Geometry: final body of the model. Coordinates: model frame, mm. Face numbers are marked on the shaded views. A direction names the side the tool comes from. Round coordinates to 2 decimals unless told otherwise and drop trailing zeros. Write each loop counter-clockwise with the first axis right and the second up, starting at its lowest first coordinate (ties: lowest second). Pieces come first, ordered by that corner, then holes. Notation, with made-up numbers: (-36.5, 81.25) -> (18.5, 81.25) arc R16 ccw to (18.5, 107.25) -> close; hole circle Ø7 at (61.5, -24). An arc over 180 degrees is marked (long way). One line per item, written item: value. Start each with the question number.
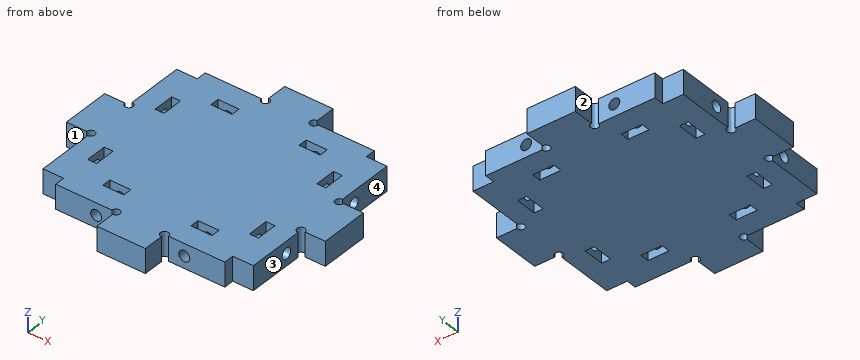
Autodesk Inventor part; units mm, degrees
ref_plane "YZ Plane" through (0, 0, 0) normal (1, 0, 0) x (0, 1, 0)
ref_plane "XZ Plane" through (0, 0, 0) normal (0, 1, 0) x (-1, 0, 0)
ref_plane "XY Plane" through (0, 0, 0) normal (0, 0, 1) x (1, 0, 0)
ref_plane "작업 평면1" through (0, 0, 0) normal (0, 0, 1) x (1, 0, 0)
sketch "스케치1" plane through (0, 0, 0) normal (0, 0, 1) x (1, 0, 0)
  line L0 (-18.9, 5.4) -> (-21.1, 5.4)
  line L1 (-21.1, 5.4) -> (-21.1, 10.6)
  line L2 (-21.1, 10.6) -> (-18.9, 10.6)
  line L3 (-18.9, 10.6) -> (-18.9, 5.4)
  line L4 (-21.1, -5.4) -> (-18.9, -5.4)
  line L5 (-18.9, -5.4) -> (-18.9, -10.6)
  line L6 (-18.9, -10.6) -> (-21.1, -10.6)
  line L7 (-21.1, -10.6) -> (-21.1, -5.4)
  line L8 (21.1, 5.4) -> (18.9, 5.4)
  line L9 (18.9, 5.4) -> (18.9, 10.6)
  line L10 (18.9, 10.6) -> (21.1, 10.6)
  line L11 (21.1, 10.6) -> (21.1, 5.4)
  line L12 (18.9, -10.6) -> (18.9, -5.4)
  line L13 (18.9, -5.4) -> (21.1, -5.4)
  line L14 (21.1, -5.4) -> (21.1, -10.6)
  line L15 (21.1, -10.6) -> (18.9, -10.6)
  circle A0 centre (8, -8) radius 1.35
  circle A1 centre (-8, 8) radius 1.35
  circle A2 centre (-8, -8) radius 1.35
  circle A3 centre (8, 8) radius 1.35
  line L16 (-26, 14) -> (-26, 3)
  line L17 (-26, 3) -> (-32, 3)
  line L18 (-32, 3) -> (-32, -3)
  line L19 (-32, -3) -> (-26, -3)
  line L20 (-26, -3) -> (-26, -14)
  line L21 (-26, -14) -> (26, -14)
  line L22 (26, -14) -> (26, -3)
  line L23 (26, -3) -> (32, -3)
  line L24 (32, -3) -> (32, 3)
  line L25 (32, 3) -> (26, 3)
  line L26 (26, 3) -> (26, 14)
  line L27 (26, 14) -> (-26, 14)
  line L28 (-11, -15.5) -> (-5, -15.5)
  line L29 (-5, -15.5) -> (-5, -18.5)
  line L30 (-5, -18.5) -> (-11, -18.5)
  line L31 (-11, -18.5) -> (-11, -15.5)
  line L32 (-5, 15.5) -> (-11, 15.5)
  line L33 (-11, 15.5) -> (-11, 18.5)
  line L34 (-11, 18.5) -> (-5, 18.5)
  line L35 (-5, 18.5) -> (-5, 15.5)
  line L36 (11, -18.5) -> (5, -18.5)
  line L37 (5, -18.5) -> (5, -15.5)
  line L38 (5, -15.5) -> (11, -15.5)
  line L39 (11, -15.5) -> (11, -18.5)
  line L40 (11, 15.0547) -> (5, 15.0547)
  line L41 (5, 15.0547) -> (5, 18.0547)
  line L42 (5, 18.0547) -> (11, 18.0547)
  line L43 (11, 18.0547) -> (11, 15.0547)
  circle A4 centre (8, 8) radius 1.35
  circle A5 centre (-8, -8) radius 1.35
  circle A6 centre (-8, 8) radius 1.35
  circle A7 centre (8, -8) radius 1.35
  line L44 (13.9, 23.5) -> (3, 23.5)
  line L45 (3, 23.5) -> (3, 29.5)
  line L46 (3, 29.5) -> (-3, 29.5)
  line L47 (-3, 29.5) -> (-3, 23.5)
  line L48 (-3, 23.5) -> (-13.9, 23.5)
  line L49 (-13.9, 23.5) -> (-13.9, -23.5)
  line L50 (-13.9, -23.5) -> (-3, -23.5)
  line L51 (-3, -23.5) -> (-3, -29.5)
  line L52 (-3, -29.5) -> (3, -29.5)
  line L53 (3, -29.5) -> (3, -23.5)
  line L54 (3, -23.5) -> (13.9, -23.5)
  line L55 (13.9, -23.5) -> (13.9, 23.5)
  line L56 (13.9, 23.5) -> (-13.9, 23.5)
  line L57 (-13.9, -23.5) -> (13.9, -23.5)
  line L58 (-26, 14) -> (-26, -14)
  line L59 (26, -14) -> (26, 14)
  line L60 (-26, -14) -> (-26, -21)
  line L61 (26, -21) -> (26, -14)
  line L62 (26, 14) -> (26, 21)
  line L63 (-26, 21) -> (-26, 14)
  line L64 (13.9, -23.5) -> (20.9, -23.5)
  line L65 (20.9, 23.5) -> (13.9, 23.5)
  line L66 (-13.9, 23.5) -> (-20.9, 23.5)
  line L67 (-20.9, -23.5) -> (-13.9, -23.5)
  line L68 (26, 21) -> (20.9, 21)
  line L69 (-20.9, 21) -> (-26, 21)
  line L70 (-20.9, -21) -> (-20.9, -23.5)
  line L71 (-20.9, 23.5) -> (-20.9, 21)
  line L72 (20.9, -23.5) -> (20.9, -21)
  line L73 (20.9, 21) -> (20.9, 23.5)
  line L74 (-26, -21) -> (-20.9, -21)
  line L75 (20.9, -21) -> (26, -21)
  line L76 (26, -5.994) -> (26, 6.006)
  line L77 (6, -23.5) -> (-6, -23.5)
  line L78 (-6, -23.5) -> (-6, -29.5)
  line L79 (-6, -29.5) -> (6, -29.5)
  line L80 (6, -29.5) -> (6, -23.5)
  line L81 (6, 23.5) -> (-6, 23.5)
  line L82 (-6, 23.5) -> (-6, 29.5)
  line L83 (-6, 29.5) -> (6, 29.5)
  line L84 (6, 29.5) -> (6, 23.5)
  line L85 (-26, 6) -> (-32, 6)
  line L86 (-32, 6) -> (-32, -6)
  line L87 (-32, -6) -> (-26, -6)
  line L88 (-26, -6) -> (-26, 6)
  line L89 (13.5, 18.1) -> (8.3, 18.1)
  line L90 (8.3, 18.1) -> (8.3, 15.9)
  line L91 (8.3, 15.9) -> (13.5, 15.9)
  line L92 (13.5, 15.9) -> (13.5, 18.1)
  line L93 (13.5, 18.1) -> (8.3, 15.9) construction
  line L94 (8.3, 18.1) -> (13.5, 15.9) construction
  line L95 (-13.5, 18.1) -> (-8.3, 18.1)
  line L96 (-8.3, 18.1) -> (-8.3, 15.9)
  line L97 (-8.3, 15.9) -> (-13.5, 15.9)
  line L98 (-13.5, 15.9) -> (-13.5, 18.1)
  line L99 (-13.5, 18.1) -> (-8.3, 15.9) construction
  line L100 (-8.3, 18.1) -> (-13.5, 15.9) construction
  line L101 (-13.5, -18.1) -> (-8.3, -18.1)
  line L102 (-8.3, -18.1) -> (-8.3, -15.9)
  line L103 (-8.3, -15.9) -> (-13.5, -15.9)
  line L104 (-13.5, -15.9) -> (-13.5, -18.1)
  line L105 (-13.5, -18.1) -> (-8.3, -15.9) construction
  line L106 (-8.3, -18.1) -> (-13.5, -15.9) construction
  line L107 (13.5, -15.9) -> (8.3, -15.9)
  line L108 (8.3, -15.9) -> (8.3, -18.1)
  line L109 (8.3, -18.1) -> (13.5, -18.1)
  line L110 (13.5, -18.1) -> (13.5, -15.9)
  line L111 (13.5, -15.9) -> (8.3, -18.1) construction
  line L112 (8.3, -15.9) -> (13.5, -18.1) construction
  line L113 (-21.1, -8) -> (-18.9, -8)
  line L114 (-18.9, -8) -> (-18.9, -13.2)
  line L115 (-18.9, -13.2) -> (-21.1, -13.2)
  line L116 (-21.1, -13.2) -> (-21.1, -8)
  line L117 (-21.1, -8) -> (-18.9, -13.2) construction
  line L118 (-18.9, -8) -> (-21.1, -13.2) construction
  line L119 (-21.1, 13.2) -> (-18.9, 13.2)
  line L120 (-18.9, 13.2) -> (-18.9, 8)
  line L121 (-18.9, 8) -> (-21.1, 8)
  line L122 (-21.1, 8) -> (-21.1, 13.2)
  line L123 (-21.1, 13.2) -> (-18.9, 8) construction
  line L124 (-18.9, 13.2) -> (-21.1, 8) construction
  line L125 (26, -5.994) -> (26, 6.006)
  line L126 (26, 6) -> (32, 6)
  line L127 (32, 6) -> (32, -6)
  line L128 (32, -6) -> (26, -6)
  line L129 (26, -6) -> (26, 6)
  line L130 (18.9, -8) -> (21.1, -8)
  line L131 (21.1, -8) -> (21.1, -13.2)
  line L132 (21.1, -13.2) -> (18.9, -13.2)
  line L133 (18.9, -13.2) -> (18.9, -8)
  line L134 (18.9, -8) -> (21.1, -13.2) construction
  line L135 (21.1, -8) -> (18.9, -13.2) construction
  line L136 (18.9, 13.2) -> (21.1, 13.2)
  line L137 (21.1, 13.2) -> (21.1, 8)
  line L138 (21.1, 8) -> (18.9, 8)
  line L139 (18.9, 8) -> (18.9, 13.2)
  line L140 (18.9, 13.2) -> (21.1, 8) construction
  line L141 (21.1, 13.2) -> (18.9, 8) construction
  point P0 (0, 0)
  point P1 (10.9, 17)
  point P2 (-10.9, 17)
  point P3 (-10.9, -17)
  point P4 (10.9, -17)
  point P5 (-20, -10.6)
  point P6 (-20, 10.6)
  point P7 (8.3, 18.0547)
  point P8 (11, 15.9)
  point P9 (-13.9, -14)
  point P10 (13.9, -14)
  point P11 (20, -10.6)
  point P12 (20, 10.6)
  dimension "d0" = 7
  dimension "d1" = 7
  dimension "d2" = 7
  dimension "d5" = 12
  dimension "d6" = 6
  dimension "d7" = 12
  dimension "d8" = 6
  dimension "d9" = 12
  dimension "d31" = 5.2
  dimension "d33" = 5.2
  dimension "d34" = 2.2
  dimension "d35" = 5.2
  dimension "d36" = 2.2
  dimension "d37" = 5.2
  dimension "d38" = 2.2
  dimension "d41" = 2.2
  dimension "d42" = 5.2
  dimension "d44" = 2.2
  dimension "d45" = 5.2
  dimension "d69" = 12
  dimension "d70" = 5.2
  dimension "d71" = 2.2
  dimension "d72" = 5.2
extrude "돌출9" add sketch "스케치1" against normal blind 6 contours L0 L1 L121 L3 | L4 L5 L113 L7 | L8 L9 L138 L11 | L12 L13 L14 L130 | A0 | A1 | A2 | A3 | L27 L49 L21 L20 L58 L16 | L63 L69 L71 L66 L49 L27 | L16 L17 L86 L85 | L49 L48 L56 L44 L55 L27 | L27 L55 L21 L49 | L58 L19 L18 L17 | L55 L65 L73 L68 L62 L27 | L27 L26 L59 L22 L21 L55 | L49 L67 L70 L74 L60 L21 | L21 L55 L54 L57 L50 L49 | L20 L87 L86 L19 | L21 L61 L75 L72 L64 L55 | L82 L83 L47 L48 | L44 L45 L83 L84 | L47 L46 L45 L56 | L50 L51 L79 L78 | L126 L127 L25 L26 | L22 L23 L127 L128 | L80 L79 L53 L54 | L57 L53 L52 L51 | L25 L24 L23 L59 | L28 L29 L30 L31 L101 L102 L103 | L32 L33 L97 L96 L95 L34 L35 | L36 L37 L38 L39 L107 L108 L109 | L40 L41 L42 L90 L91 L43
sketch "스케치7" plane through (-32, -6, 0) normal (-1, 0, 0) x (0, 0, 1)
  line L0 (0, 19.2) -> (0, 14)
  circle A0 centre (-3, 16.6) radius 1.35
  line L1 (0, -2) -> (0, -7.2)
  circle A1 centre (-3, -4.6) radius 1.35
  point P0 (0, 6)
  dimension "d75" = 2.7
  dimension "d76" = 2.7
extrude "돌출10" cut sketch "스케치7" against normal blind 16
sketch "스케치8" plane through (32, -6, 0) normal (1, 0, 0) x (0, 0, -1)
  line L0 (6, 19.2) -> (6, 14)
  line L1 (6, -2) -> (6, -7.2)
  circle A0 centre (3, 16.6) radius 1.35
  circle A1 centre (3, -4.6) radius 1.35
  point P0 (0, 6)
  dimension "d79" = 2.7
  dimension "d80" = 2.7
extrude "돌출11" cut sketch "스케치8" against normal blind 16
sketch "스케치9" plane through (-6, -29.5, 0) normal (0, -1, 0) x (1, 0, 0)
  line L0 (19.5, -6) -> (14.3, -6)
  line L1 (-2.3, -6) -> (-7.5, -6)
  circle A0 centre (16.9, -3) radius 1.35
  circle A1 centre (-4.9, -3) radius 1.35
  point P0 (6, 0)
  dimension "d83" = 2.7
  dimension "d84" = 2.7
extrude "돌출12" cut sketch "스케치9" against normal blind 16
sketch "스케치10" plane through (-6, 29.5, 0) normal (0, 1, 0) x (1, 0, 0)
  line L0 (19.5, 0) -> (14.3, 0)
  line L1 (-2.3, 0) -> (-7.5, 0)
  circle A0 centre (-4.9, 3) radius 1.35
  circle A1 centre (16.9, 3) radius 1.35
  point P0 (6, 0)
  dimension "d87" = 2.7
  dimension "d88" = 2.7
extrude "돌출13" cut sketch "스케치10" against normal blind 16
sketch "스케치11" plane through (0, 0, 0) normal (0, 0, 1) x (1, 0, 0)
  line L0 (-6, -29.5) -> (6, -29.5)
  line L1 (6, -29.5) -> (6, -23.5)
  line L2 (6, -23.5) -> (20.9, -23.5)
  line L3 (20.9, -23.5) -> (20.9, -21)
  line L4 (20.9, -21) -> (26, -21)
  line L5 (26, -21) -> (26, -6)
  line L6 (26, -6) -> (32, -6)
  line L7 (32, -6) -> (32, 6)
  line L8 (32, 6) -> (26, 6)
  line L9 (26, 6) -> (26, 21)
  line L10 (26, 21) -> (20.9, 21)
  line L11 (20.9, 21) -> (20.9, 23.5)
  line L12 (20.9, 23.5) -> (6, 23.5)
  line L13 (6, 23.5) -> (6, 29.5)
  line L14 (6, 29.5) -> (-6, 29.5)
  line L15 (-6, 29.5) -> (-6, 23.5)
  line L16 (-6, 23.5) -> (-20.9, 23.5)
  line L17 (-20.9, 23.5) -> (-20.9, 21)
  line L18 (-20.9, 21) -> (-26, 21)
  line L19 (-26, 21) -> (-26, 6)
  line L20 (-26, 6) -> (-32, 6)
  line L21 (-32, 6) -> (-32, -6)
  line L22 (-32, -6) -> (-26, -6)
  line L23 (-26, -6) -> (-26, -21)
  line L24 (-26, -21) -> (-20.9, -21)
  line L25 (-20.9, -21) -> (-20.9, -23.5)
  line L26 (-20.9, -23.5) -> (-6, -23.5)
  line L27 (-6, -23.5) -> (-6, -29.5)
  line L28 (8.3, -15.9) -> (13.5, -15.9)
  line L29 (13.5, -15.9) -> (13.5, -18.1)
  line L30 (13.5, -18.1) -> (8.3, -18.1)
  line L31 (8.3, -18.1) -> (8.3, -15.9)
  line L32 (-8.3, -18.1) -> (-13.5, -18.1)
  line L33 (-13.5, -18.1) -> (-13.5, -15.9)
  line L34 (-13.5, -15.9) -> (-8.3, -15.9)
  line L35 (-8.3, -15.9) -> (-8.3, -18.1)
  line L36 (-18.9, -8) -> (-18.9, -13.2)
  line L37 (-18.9, -13.2) -> (-21.1, -13.2)
  line L38 (-21.1, -13.2) -> (-21.1, -8)
  line L39 (-21.1, -8) -> (-18.9, -8)
  line L40 (-21.1, 8) -> (-21.1, 13.2)
  line L41 (-21.1, 13.2) -> (-18.9, 13.2)
  line L42 (-18.9, 13.2) -> (-18.9, 8)
  line L43 (-18.9, 8) -> (-21.1, 8)
  line L44 (-8.3, 15.9) -> (-13.5, 15.9)
  line L45 (-13.5, 15.9) -> (-13.5, 18.1)
  line L46 (-13.5, 18.1) -> (-8.3, 18.1)
  line L47 (-8.3, 18.1) -> (-8.3, 15.9)
  line L48 (8.3, 15.9) -> (8.3, 18.1)
  line L49 (8.3, 18.1) -> (13.5, 18.1)
  line L50 (13.5, 18.1) -> (13.5, 15.9)
  line L51 (13.5, 15.9) -> (8.3, 15.9)
  line L52 (18.9, 8) -> (18.9, 13.2)
  line L53 (18.9, 13.2) -> (21.1, 13.2)
  line L54 (21.1, 13.2) -> (21.1, 8)
  line L55 (21.1, 8) -> (18.9, 8)
  line L56 (21.1, -8) -> (21.1, -13.2)
  line L57 (21.1, -13.2) -> (18.9, -13.2)
  line L58 (18.9, -13.2) -> (18.9, -8)
  line L59 (18.9, -8) -> (21.1, -8)
  circle A0 centre (26, 6) radius 1
  circle A1 centre (26, -6) radius 1
  circle A2 centre (6, -23.5) radius 1
  circle A3 centre (-6, -23.5) radius 1
  circle A4 centre (-26, -6) radius 1
  circle A5 centre (-26, 6) radius 1
  circle A6 centre (-6, 23.5) radius 1
  circle A7 centre (6, 23.5) radius 1
  point P0 (0, 0)
  dimension "d91" = 2
  dimension "d92" = 2
  dimension "d93" = 2
  dimension "d94" = 2
  dimension "d95" = 2
  dimension "d96" = 2
  dimension "d97" = 2
  dimension "d98" = 2
extrude "돌출14" cut sketch "스케치11" against normal blind 10 contours A3 L26 L27 | L27 L26 A3 | A2 L2 L1 | L1 L2 A2 | A4 L22 L23 | L23 L22 A4 | A1 L6 L5 | L5 L6 A1 | A5 L19 L20 | L20 L19 A5 | A0 L9 L8 | L8 L9 A0 | A6 L15 L16 | L16 L15 A6 | A7 L13 L12 | L12 L13 A7
properties part number "connection_leg_ver2" material "PMMA 플라스틱"
(1) Pin query (flat end, axial travel): pin 1 (0.7 mm diameter, centred on x = -20, z = -4, fed in from -Y); pin 2 (1.1 mm diameter, centred on x = 19.5, z = -2.5, fed in from +Y); pin 3 (3 mm diameter, centred on y = 10.6, z = -3, fed in from +X). Return the tip coordinate at first contact, or that it passes through.
(2) Section query B-B (x = 10.9). Output: boundary loops of the cut face in (y, z), and give its area (3 significant figures).
(3) Section query C-C (z = -5.3). Count the separate pieces of the cut face and the enclosed holes in it, and give its area (3 significant figures).
(4) Set-up query: the marked faces 1, 2, 3 and 4. Return all of +Z, -Z, +X, -X, +Y, -Y with unobstructed straight access to the full face (end or side cutting, diameter ignored); none if empty.
(5) Section query A-A (y = 10.6). Output: boundary loops of the cut face in (x, z).
(6) Line query: probe 1 along Y at (x, z) = (-10.5, -5.6); probe 2 along X at (y, z) = (20.1, -3); probe 3 along X at (y, z) = (13, -1.2). Output: solid intervals per line, ascending.
Results list:
1. pin 1: stops at y = -23.5
1. pin 2: stops at y = 23.5
1. pin 3: stops at x = 26
2. outline: (-23.5, -6) -> (-18.1, -6) -> (-18.1, -4.35) -> (-23.5, -4.35) -> close; (-23.5, -1.65) -> (-18.1, -1.65) -> (-18.1, 0) -> (-23.5, 0) -> close; (-15.9, -6) -> (15.9, -6) -> (15.9, -4.35) -> (13.5, -4.35) -> (13.5, -1.65) -> (15.9, -1.65) -> (15.9, 0) -> (-15.9, 0) -> (-15.9, -1.65) -> (-13.5, -1.65) -> (-13.5, -4.35) -> (-15.9, -4.35) -> close; (18.1, -6) -> (23.5, -6) -> (23.5, -4.35) -> (18.1, -4.35) -> close; (18.1, -1.65) -> (23.5, -1.65) -> (23.5, 0) -> (18.1, 0) -> close
2. area: 213 mm^2
3. separate pieces: 1
3. enclosed holes: 8
3. area: 2,570 mm^2
4. face 1: +Z, -Z, -X, -Y
4. face 2: +Z, -Z, -X, +Y
4. face 3: +Z, -Z, +X, -Y
4. face 4: +Z, -Z, +X, +Y
5. outline: (-26, -6) -> (-21.1, -6) -> (-21.1, -4.35) -> (-26, -4.35) -> close; (-26, -1.65) -> (-21.1, -1.65) -> (-21.1, 0) -> (-26, 0) -> close; (-18.9, -6) -> (18.9, -6) -> (18.9, -4.35) -> (16, -4.35) -> (16, -1.65) -> (18.9, -1.65) -> (18.9, 0) -> (-18.9, 0) -> (-18.9, -1.65) -> (-16, -1.65) -> (-16, -4.35) -> (-18.9, -4.35) -> close; (21.1, -6) -> (26, -6) -> (26, -4.35) -> (21.1, -4.35) -> close; (21.1, -1.65) -> (26, -1.65) -> (26, 0) -> (21.1, 0) -> close
6. probe 1: y = -23.5 to -18.1, -15.9 to 15.9, 18.1 to 23.5
6. probe 2: x = -26 to -12.25, -9.55 to 9.55, 12.25 to 26
6. probe 3: x = -26 to -21.1, -18.9 to 18.9, 21.1 to 26
